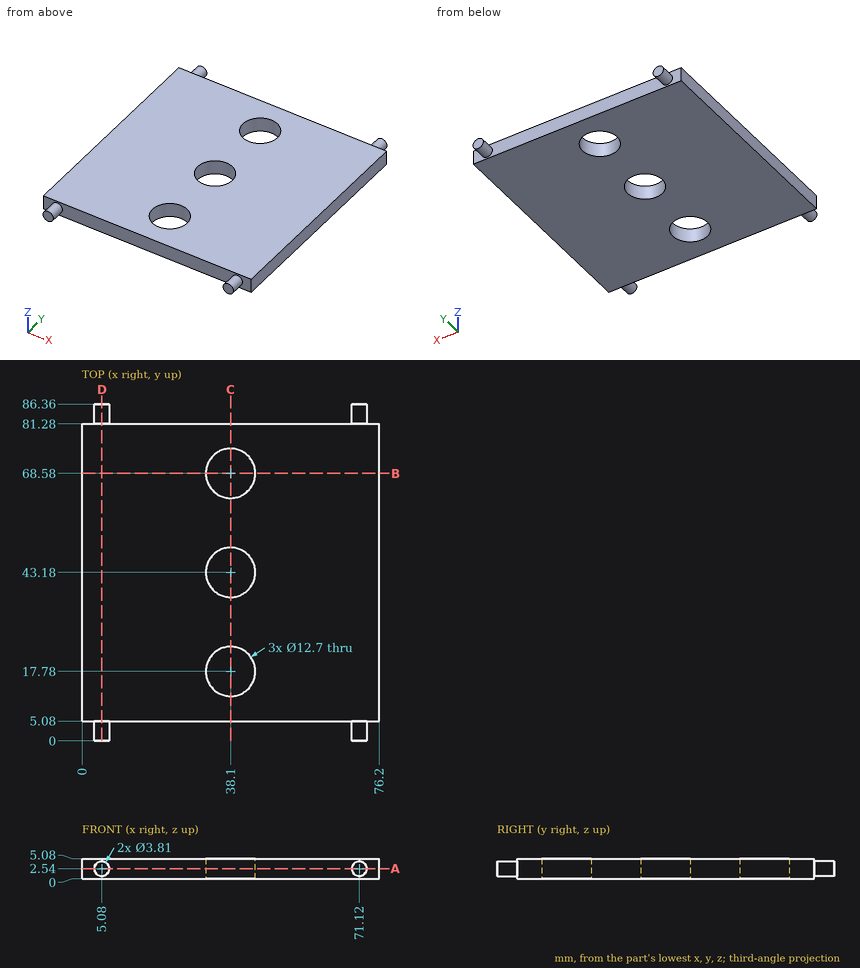
Study the drawing (mm; zero at the part's minimum x, y, z) and answer. Give positions to 0.01 mm unless a question says otherwise; leave off trailing zeros. Write each loop counter-clockwise with the first axis right and the second up, starting at its lowest first coordinate (ties: lowest second). Pieces come first, ordered by that corner, then holes. Notation, with made-up numbers: (-1.5, -36.5) -> (15.5, -36.5) arc R23 ccw to (15.5, -28.5) -> close; hole circle Ø11 at (35, -39.5). An arc over 180 degrees is marked (long way). Answer in a Markdown table with one row per item.
1) Each of these flat-tipped pins is pushed along its axis until it touches: pin 1 Ø4 at (x, y) = (43, 72) entering from -Z; pin 2 Ø7.5 at (x, y) = (38.1, 43.18) entering from -Z; pin 3 Ø2 at (x, z) = (11.5, 1) entering from +Y. Where does it stop, or does it pass through?
Results list:
| item | result |
|---|---|
| pin 1 | z = 0 |
| pin 2 | through |
| pin 3 | y = 81.28 |
2) Section D-D on x = 5.08 is taken. Give the vertices of the cut face in (y, z) (3 decimals), plus the area to 3 significant figures.
Results list:
| item | result |
|---|---|
| outline | (0, 0.635) -> (5.08, 0.635) -> (5.08, 0) -> (81.28, 0) -> (81.28, 0.635) -> (86.36, 0.635) -> (86.36, 4.445) -> (81.28, 4.445) -> (81.28, 5.08) -> (5.08, 5.08) -> (5.08, 4.445) -> (0, 4.445) -> close |
| area | 426 mm^2 |
3) Section C-C on x = 38.1 is taken. Give the vertices of the cut face in (y, z).
Results list:
| item | result |
|---|---|
| outline | (5.08, 0) -> (11.43, 0) -> (11.43, 5.08) -> (5.08, 5.08) -> close; (24.13, 0) -> (36.83, 0) -> (36.83, 5.08) -> (24.13, 5.08) -> close; (49.53, 0) -> (62.23, 0) -> (62.23, 5.08) -> (49.53, 5.08) -> close; (74.93, 0) -> (81.28, 0) -> (81.28, 5.08) -> (74.93, 5.08) -> close |
4) Section B-B on y = 68.58 is taken. Give the vertices of the cut face in (x, z).
Results list:
| item | result |
|---|---|
| outline | (0, 0) -> (31.75, 0) -> (31.75, 5.08) -> (0, 5.08) -> close; (44.45, 0) -> (76.2, 0) -> (76.2, 5.08) -> (44.45, 5.08) -> close |
5) Straight lines are drawn through the part: line 1 (Y direction, x = 38.1, z = 3.65); line 2 (X direction, y = 81.5, z = 2.6); line 3 (Y direction, x = 68, z = 1.7). For each, find the intervals that lie inside material, in ascending order. Write a range as [from, to].
Results list:
| item | result |
|---|---|
| line 1 | [5.08, 11.43], [24.13, 36.83], [49.53, 62.23], [74.93, 81.28] |
| line 2 | [3.18, 6.98], [69.22, 73.02] |
| line 3 | [5.08, 81.28] |
6) Section A-A on z = 2.54 is taken. Give the vertices of the cut face in (x, y) (3 decimals), plus the area to 3 significant figures.
Results list:
| item | result |
|---|---|
| outline | (0, 5.08) -> (3.175, 5.08) -> (3.175, 0) -> (6.985, 0) -> (6.985, 5.08) -> (69.215, 5.08) -> (69.215, 0) -> (73.025, 0) -> (73.025, 5.08) -> (76.2, 5.08) -> (76.2, 81.28) -> (73.025, 81.28) -> (73.025, 86.36) -> (69.215, 86.36) -> (69.215, 81.28) -> (6.985, 81.28) -> (6.985, 86.36) -> (3.175, 86.36) -> (3.175, 81.28) -> (0, 81.28) -> close; hole circle Ø12.7 at (38.1, 17.78); hole circle Ø12.7 at (38.1, 43.18); hole circle Ø12.7 at (38.1, 68.58) |
| area | 5,500 mm^2 |
